```python
from build123d import *

# Parameters (mm, degrees)
F0_R     = 6.35
F1_DEPTH = 38.1
F3_R     = 5.3975
F4_DEPTH = 32.512
F5_R     = 12.7
F6_DEPTH = 6.858
F2_R     = 1.778
F7_DEPTH = 50.292


with BuildPart() as f1:
    # F0 (on Top) → F1 (new body)
    with BuildSketch(Plane.XY):
        Circle(F0_R)
    extrude(amount=F1_DEPTH)

    # F3 (on face) → F4 (cut)
    with BuildSketch(Plane(origin=(0, 0, 0), x_dir=(1, 0, 0), z_dir=(0, 0, -1))):
        Circle(F3_R)
    extrude(amount=-F4_DEPTH, mode=Mode.SUBTRACT)

    # F5 (on face) → F6 (join)
    with BuildSketch(Plane.XY.offset(38.1)):
        Circle(F5_R)
    extrude(amount=-F6_DEPTH)

    # F2 (on face) → F7 (cut)
    with BuildSketch(Plane(origin=(0, 0, 0), x_dir=(1, 0, 0), z_dir=(0, 0, -1))):
        Circle(F2_R)
    extrude(amount=-F7_DEPTH, mode=Mode.SUBTRACT)


solid = f1.part
```
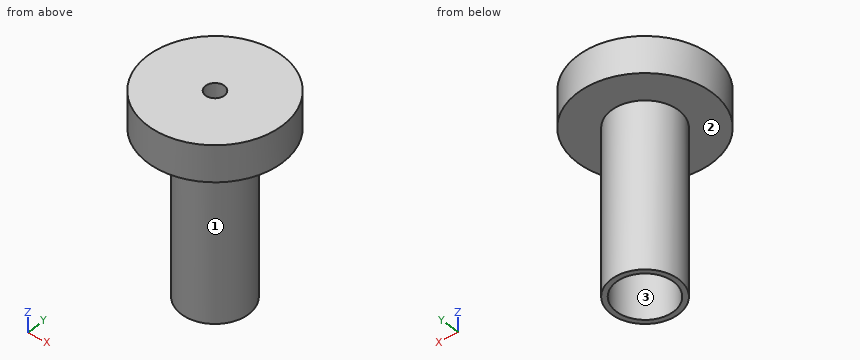
Source: CAD feature listing. Evaluate the final solid. Frame: model axes, mm. Face numbers are marked on the shaded views. Give positions to 0.01 mm unless a question says otherwise; leave off trailing zeros. Order: outer loops, then holes, each group sorted by start corner. A loop starts at its lowest first (then second) coordinate and runs counter-clockwise, first axis right, second up. Notation, with made-up numbers: (50, -2.5) -> (82, -2.5) arc R21 ccw to (82, 31.5) -> close; hole circle Ø3 at (82.25, 8.25). An arc over 180 degrees is marked (long way). Use a Markdown table: item, result.
Q1. Section A-A (y = 0). Return the cut outline in (x, z).
A:
| item | result |
|---|---|
| outline | (-12.7, 31.24) -> (-6.35, 31.24) -> (-6.35, 0) -> (-5.4, 0) -> (-5.4, 31.24) -> (-1.78, 31.24) -> (-1.78, 38.1) -> (-12.7, 38.1) -> close; (1.78, 31.24) -> (5.4, 31.24) -> (5.4, 0) -> (6.35, 0) -> (6.35, 31.24) -> (12.7, 31.24) -> (12.7, 38.1) -> (1.78, 38.1) -> close |
Q2. First-contact query: P1, Ø6, axis at x = 3.5, z = 11.5, coming from the -Y side; P2, Ø12, axis at x = -6, y = -6.5, coming from the -Z side; P3, Ø1.5, axis at x = -5.5, z = 25, coming from the -Y side; P4, Ø10, axis at y = 0.5, z = 17.5, coming from the +X side. Flat tips, straight axial feed; report the tip coordinate or a pass-through.
A:
| item | result |
|---|---|
| P1 | y = -6.33 |
| P2 | z = 0 |
| P3 | y = -4.21 |
| P4 | x = 6.35 |
Q3. Material intervals for line 1 (X direction, y = 0, z = 22); line 2 (Z direction, x = -7.5, y = 8.25), sorted ascending. Write a range as [from, to].
A:
| item | result |
|---|---|
| line 1 | [-6.35, -5.4], [5.4, 6.35] |
| line 2 | [31.24, 38.1] |
Q4. Pull-direction query (X, two-part tool) for the marked faces 1, 2 and 3; classes: +X half, -X half, draft (parallel to the pull), parting line (faces both ways), or undercut.
A:
| item | result |
|---|---|
| face 1 | parting line |
| face 2 | draft |
| face 3 | undercut |
Q5. Section D-D (x = -3.5). Return the cut outline in (y, z).
A:
| item | result |
|---|---|
| outline | (-12.21, 31.24) -> (-5.3, 31.24) -> (-5.3, 0) -> (-4.11, 0) -> (-4.11, 31.24) -> (4.11, 31.24) -> (4.11, 0) -> (5.3, 0) -> (5.3, 31.24) -> (12.21, 31.24) -> (12.21, 38.1) -> (-12.21, 38.1) -> close |
